from build123d import *

# Parameters (mm, degrees)
EXTRUDE_2_DEPTH      = 5
EXTRUDE_3_DEPTH      = 23.5
SKETCH_3_R           = 1.65
CUT_EXTRUDE_1_DEPTH  = 85.951456727
CUT_EXTRUDE_5_REACH  = 89.951
CUT_EXTRUDE_START    = 3
SKETCH_8_R           = 3
CUT_EXTRUDE_10_REACH = 89.951
CUT_EXTRUDE_START_2  = -3
SKETCH_12_R          = 3
SKETCH_4_W           = 20
SKETCH_4_H           = 10
CUT_EXTRUDE_2_DEPTH  = 5
SKETCH_10_W          = 16
SKETCH_10_H          = 40
CUT_EXTRUDE_11_DEPTH = 85.951456727
FILLET_1_R           = 3
CUT_EXTRUDE_6_DEPTH  = 94.465851734
SKETCH_6_R           = 2.6
CUT_EXTRUDE_3_DEPTH  = 83.421182124
CUT_EXTRUDE_4_REACH  = 89.421
CUT_EXTRUDE_START_3  = -5
SKETCH_7_R           = 4.4
FILLET_3_R           = 2


with BuildPart() as part:
    # 草图2 → 凸台-拉伸2 (new body)
    with BuildSketch(Plane(origin=(0, 0, 0), x_dir=(1, 0, 0), z_dir=(0, 1, 0))):
        Polygon((0, 0), (23.5, 0), (23.5, -19), (23.5, -80), (0, -80), align=None)
    extrude_2 = extrude(amount=EXTRUDE_2_DEPTH)

    # 镜向1: 凸台-拉伸2 across plane
    add(extrude_2.mirror(Plane(origin=(0, 5, 80), x_dir=(0, 0, 1), z_dir=(1, 0, 0))))

    # 草图5 → 凸台-拉伸3 (add, symmetric)
    with BuildSketch(Plane(origin=(0, 0, 0), x_dir=(0, 0, -1), z_dir=(1, 0, 0))):
        Polygon((-80, 0), (-16.263455967, -11.263455967), (-11.242997821, -6.242997821), (-10.88944443, -6.596551211), (-6.788225099, -2.495331881), (-7.14177849, -2.14177849), (-5, 0), align=None)
    extrude(amount=EXTRUDE_3_DEPTH, both=True)

    # 草图3 → 切除-拉伸1 (cut, through all)
    with BuildSketch(Plane(origin=(0, 5, 0), x_dir=(1, 0, 0), z_dir=(0, 1, 0))):
        with Locations(Location((-20, -20, 0), (0, 0, 270))):
            Circle(SKETCH_3_R)
        with Locations(Location((20, -20, 0), (0, 0, 270))):
            Circle(SKETCH_3_R)
        with Locations(Location((-20, -75, 0), (0, 0, 270))):
            Circle(SKETCH_3_R)
        with Locations(Location((20, -75, 0), (0, 0, 270))):
            Circle(SKETCH_3_R)
    extrude(amount=-CUT_EXTRUDE_1_DEPTH, mode=Mode.SUBTRACT)

    # 切除-拉伸5: up to this plane
    cut_extrude_5_end = Plane(origin=(23.5, -13.709378738, 2.422707194), z_dir=(0, 0.9847416717466503, -0.174022527063632))
    # 草图8 → 切除-拉伸5 (cut, up to the surface)
    with BuildSketch(Plane.XZ.offset(-5).offset(CUT_EXTRUDE_START), mode=Mode.PRIVATE) as cut_extrude_5_sk1:
        with Locations(Location((-20, 20, 0), (0, 0, 90))):
            Circle(SKETCH_8_R)
    cut_extrude_5_tool1 = split(extrude(cut_extrude_5_sk1.sketch, amount=CUT_EXTRUDE_5_REACH, mode=Mode.PRIVATE), bisect_by=cut_extrude_5_end, keep=Keep.BOTH, mode=Mode.PRIVATE)
    add(cut_extrude_5_tool1.solids().sort_by_distance((-20, 2, 20))[0], mode=Mode.SUBTRACT)
    # 草图8 → 切除-拉伸5 (cut, up to the surface)
    with BuildSketch(Plane.XZ.offset(-5).offset(CUT_EXTRUDE_START), mode=Mode.PRIVATE) as cut_extrude_5_sk2:
        with Locations(Location((20, 20, 0), (0, 0, 90))):
            Circle(SKETCH_8_R)
    cut_extrude_5_tool2 = split(extrude(cut_extrude_5_sk2.sketch, amount=CUT_EXTRUDE_5_REACH, mode=Mode.PRIVATE), bisect_by=cut_extrude_5_end, keep=Keep.BOTH, mode=Mode.PRIVATE)
    add(cut_extrude_5_tool2.solids().sort_by_distance((20, 2, 20))[0], mode=Mode.SUBTRACT)

    # 切除-拉伸10: up to this plane
    cut_extrude_10_end = Plane(origin=(23.5, -13.709378738, 2.422707194), z_dir=(0, 0.9847416717466503, -0.174022527063632))
    # 草图12 → 切除-拉伸10 (cut, up to the surface)
    with BuildSketch(Plane(origin=(0, 5, 0), x_dir=(1, 0, 0), z_dir=(0, 1, 0)).offset(CUT_EXTRUDE_START_2), mode=Mode.PRIVATE) as cut_extrude_10_sk1:
        with Locations(Location((-20, -75, 0), (0, 0, 270))):
            Circle(SKETCH_12_R)
    cut_extrude_10_tool1 = split(extrude(cut_extrude_10_sk1.sketch, amount=-CUT_EXTRUDE_10_REACH, mode=Mode.PRIVATE), bisect_by=cut_extrude_10_end, keep=Keep.BOTH, mode=Mode.PRIVATE)
    add(cut_extrude_10_tool1.solids().sort_by_distance((-20, 2, 75))[0], mode=Mode.SUBTRACT)
    # 草图12 → 切除-拉伸10 (cut, up to the surface)
    with BuildSketch(Plane(origin=(0, 5, 0), x_dir=(1, 0, 0), z_dir=(0, 1, 0)).offset(CUT_EXTRUDE_START_2), mode=Mode.PRIVATE) as cut_extrude_10_sk2:
        with Locations(Location((20, -75, 0), (0, 0, 270))):
            Circle(SKETCH_12_R)
    cut_extrude_10_tool2 = split(extrude(cut_extrude_10_sk2.sketch, amount=-CUT_EXTRUDE_10_REACH, mode=Mode.PRIVATE), bisect_by=cut_extrude_10_end, keep=Keep.BOTH, mode=Mode.PRIVATE)
    add(cut_extrude_10_tool2.solids().sort_by_distance((20, 2, 75))[0], mode=Mode.SUBTRACT)

    # 草图4 → 切除-拉伸2 (cut)
    with BuildSketch(Plane(origin=(0, 5, 0), x_dir=(1, 0, 0), z_dir=(0, 1, 0))):
        with Locations((0, -16)):
            Rectangle(SKETCH_4_W, SKETCH_4_H)
    extrude(amount=-CUT_EXTRUDE_2_DEPTH, mode=Mode.SUBTRACT)

    # 草图10 → 切除-拉伸11 (cut, through all)
    with BuildSketch(Plane(origin=(0, 5, 0), x_dir=(1, 0, 0), z_dir=(0, 1, 0))):
        with Locations((0, -42)):
            Rectangle(SKETCH_10_W, SKETCH_10_H)
        Polygon((-7, -72), (-15, -80), (15, -80), (7, -72), align=None)
        Polygon((23.5, -22), (15.5, -26.618802154), (15.5, -68.269538735), (23.5, -72), align=None)
        Polygon((-15.5, -26.618802154), (-23.5, -22), (-23.5, -72), (-15.5, -68.269538735), align=None)
    extrude(amount=-CUT_EXTRUDE_11_DEPTH, mode=Mode.SUBTRACT)

    # 圆角1
    fillet_1_edges = [part.edges().sort_by_distance(p)[0] for p in [
        (-23.5, -2.624849927, 22),
        (-23.5, 1.793124148, 72),
        (23.5, 1.793124148, 72),
        (23.5, -2.624849927, 22),
        (15, 2.5, 80),
        (-15, 2.5, 80),
        (-15.5, -2.216734964, 26.618802154),
        (-15.5, 1.463502525, 68.269538735),
        (15.5, 1.463502525, 68.269538735),
        (15.5, -2.216734964, 26.618802154),
        (-7, 1.793124148, 72),
        (7, 1.793124148, 72),
        (-23.5, 2.5, 80),
        (23.5, 2.5, 80),
    ]]
    fillet(fillet_1_edges, radius=FILLET_1_R)

    # 草图9 → 切除-拉伸6 (cut, through all)
    with BuildSketch(Plane(origin=(23.5, 0, 0), x_dir=(0, 0, -1), z_dir=(1, 0, 0))):
        Polygon((-5, 0), (0, 5), (0, 0), align=None)
    extrude(amount=-CUT_EXTRUDE_6_DEPTH, mode=Mode.SUBTRACT)

    # 草图6 → 切除-拉伸3 (cut, through all)
    with BuildSketch(Plane(origin=(0, 2.146446609, 2.146446609), x_dir=(1, 0, 0), z_dir=(0, -0.7071067811865459, -0.7071067811865491))):
        with Locations(Location((-13.5, 9.464466094, 0), (0, 0, 270))):
            Circle(SKETCH_6_R)
        with Locations(Location((13.5, 9.464466094, 0), (0, 0, 270))):
            Circle(SKETCH_6_R)
    extrude(amount=-CUT_EXTRUDE_3_DEPTH, mode=Mode.SUBTRACT)

    # 草图7 → 切除-拉伸4 (cut, up to next)
    with BuildSketch(Plane(origin=(0, 2.146446609, 2.146446609), x_dir=(1, 0, 0), z_dir=(0, -0.7071067811865459, -0.7071067811865491)).offset(CUT_EXTRUDE_START_3), mode=Mode.PRIVATE) as cut_extrude_4_sk1:
        with Locations((-13.5, 9.464466094)):
            Circle(SKETCH_7_R)
    cut_extrude_4_tool1 = extrude(cut_extrude_4_sk1.sketch, amount=-CUT_EXTRUDE_4_REACH, mode=Mode.PRIVATE) & part.part
    # 草图7 → 切除-拉伸4 (cut, up to next)
    with BuildSketch(Plane(origin=(0, 2.146446609, 2.146446609), x_dir=(1, 0, 0), z_dir=(0, -0.7071067811865459, -0.7071067811865491)).offset(CUT_EXTRUDE_START_3), mode=Mode.PRIVATE) as cut_extrude_4_sk2:
        with Locations((13.5, 9.464466094)):
            Circle(SKETCH_7_R)
    cut_extrude_4_tool2 = extrude(cut_extrude_4_sk2.sketch, amount=-CUT_EXTRUDE_4_REACH, mode=Mode.PRIVATE) & part.part
    add(cut_extrude_4_tool1.solids().sort_by_distance((-13.5, -1.010408, 12.374369))[0], mode=Mode.SUBTRACT)
    add(cut_extrude_4_tool2.solids().sort_by_distance((13.5, -1.010408, 12.374369))[0], mode=Mode.SUBTRACT)

    # 圆角3
    fillet_3_edges = [part.edges().sort_by_distance(p)[0] for p in [
        (0, 5, 0),
    ]]
    fillet(fillet_3_edges, radius=FILLET_3_R)


solid = part.part
Can you work these out from the model? Positions are in its coordinate system, mm. A direction names the side the tool comes from. Give positions to 0.01 mm unless a question says otherwise; leave off trailing zeros. Loops run counter-clockwise (first coordinate to the right, second up) from the corner with the lowest first, then second, coordinate; pieces in that order, holes last. Notation, with made-up numbers: (23.5, 51.5) -> (36.5, 51.5) arc R22 ccw to (36.5, 58.5) -> close; hole circle Ø2 at (41, -12.75). An arc over 180 degrees is marked (long way). Write item = value, one per line.
1) I need wall thicknesses on L1, parallel to X at y = 0.8, z = 75; L2, parallel to X at y = -2.25, z = 20; L3, parallel to Z at x = -20, y = -0.65. Which ranges of each line are inside material? Lowest first, please. Write a range as from..to.
Check result:
L1 = -23.5..-23, -17..-10, 10..17, 23..23.5
L2 = -23.5..-23, -17..17, 23..23.5
L3 = 5.65..17, 23..24.02, 70.37..72
2) Suppose I cut it at B-B on z = 50.5. Write out the boundary of the cut face in (x, y), then the cut area to 3 significant figures.
Check result:
outline = (-15.5, -5.21) -> (-8, -5.21) -> (-8, 5) -> (-15.5, 5) -> close; (8, -5.21) -> (15.5, -5.21) -> (15.5, 5) -> (8, 5) -> close
area = 153 mm2
3) Thinking about a two-plate mould opening in Z: for faces 6 (the flat face through (23.5, -1, 14)), 7 (the flat face through (11, 2, 76)), 8 (the cylindrical face through (-15.957, 1.243, 67.95)), which applies, released by +Z, released by -Z, zero draft, split by the parting line, or undercut?
Check result:
face_6 = zero draft
face_7 = released by +Z
face_8 = undercut
4) For faces 1 (the cylindrical face through (-23.11, -2.89, 21.75)), 2 (the flat face through (0, 3, 11)), 3 (the flat face through (0, -3, 22)), 4 (the cylindrical face through (15.983, 1.243, 67.99)), 5 (the cylindrical face through (-6.921, 1.748, 72.235)), which set-ups out of +Z, -Z, +X, -X, +Y, -Y let a thin tool reach every point of the face, with its end or its side?
Check result:
face_1 = -X, +Y, -Y
face_2 = +Y
face_3 = +Y, -Y
face_4 = +X, +Y, -Y
face_5 = +Z, +Y, -Y
5) Suppose I cut it at A-A on x = -1. Write out the boundary of the cut face in (y, z).
Check result:
outline = (-11.26, 16.26) -> (-6.24, 11.24) -> (-6.6, 10.89) -> (-2.5, 6.79) -> (-2.14, 7.14) -> (1.59, 3.41) arc R2 ccw to (5, 4.83) -> (5, 11) -> (0, 11) -> (0, 21) -> (5, 21) -> (5, 22) -> (-10.25, 22) -> close; (-3.18, 62) -> (5, 62) -> (5, 72) -> (-1.41, 72) -> close
6) Suppose I cut it at D-D on z = 30.5. Write out the boundary of the cut face in (x, y).
Check result:
outline = (-15.5, -8.75) -> (-8, -8.75) -> (-8, 5) -> (-15.5, 5) -> close; (8, -8.75) -> (15.5, -8.75) -> (15.5, 5) -> (8, 5) -> close
7) Will these pins go through, and if not, where does the flat tip stop? pin 1 (2.5 mm diameter, centred on x = 3, y = 2.5, fed in from -Z); pin 2 (3 mm diameter, centred on x = 20, z = 76, fed in from -Y); pin 3 (4 mm diameter, centred on x = -19, z = 71.5, fed in from -Y); pin 4 (2 mm diameter, centred on x = -15, y = -1.5, fed in from -Z).
Check result:
pin_1 = 2.83
pin_2 = 2
pin_3 = -1.84
pin_4 = 5.5
8) Suppose I cut it at C-C on z = 75. Write out the boundary of the cut face in (x, y).
Check result:
outline = (-23.5, -0.88) -> (-23, -0.88) -> (-23, 2) -> (-21.65, 2) -> (-21.65, 5) -> (-23.5, 5) -> close; (-18.35, 2) -> (-17, 2) -> (-17, -0.88) -> (-10, -0.88) -> (-10, 5) -> (-18.35, 5) -> close; (10, -0.88) -> (17, -0.88) -> (17, 2) -> (18.35, 2) -> (18.35, 5) -> (10, 5) -> close; (21.65, 2) -> (23, 2) -> (23, -0.88) -> (23.5, -0.88) -> (23.5, 5) -> (21.65, 5) -> close
